from build123d import *

# Parameters (mm, degrees)
SKIZZE1_W                       = 72
SKIZZE1_H                       = 44.2
SKIZZE1_R                       = 10
SKIZZE1_R_2                     = 6
AUFSATZ_LINEAR_AUSTRAGEN1_DEPTH = 20
FASE1_SIZE                      = 10
FASE2_SIZE                      = 10
FASE6_SIZE                      = 10
FASE6_SIZE2                     = 3.639702343
FASE7_SIZE                      = 5
SKIZZE3_W                       = 5
SKIZZE3_H                       = 17
SCHNITT_LINEAR_AUSTRAGEN1_DEPTH = 80
SKIZZE11_R                      = 12
SCHNITT_LINEAR_AUSTRAGEN2_DEPTH = 3.4
M5_GEWINDEBOHRUNG1_D            = 4.2
M5_GEWINDEBOHRUNG1_DEPTH        = 12
M5_GEWINDEBOHRUNG1_TIP          = 1.2618073


with BuildPart() as part:
    # Skizze1 → Aufsatz-Linear austragen1 (new body)
    with BuildSketch(Plane.XY):
        with Locations((53.961300324, 0)):
            Rectangle(SKIZZE1_W, SKIZZE1_H)
        with Locations((53.961300324, -9.9)):
            Circle(SKIZZE1_R, mode=Mode.SUBTRACT)
        with Locations((33.961300324, -9.9)):
            Circle(SKIZZE1_R_2, mode=Mode.SUBTRACT)
        with Locations((73.961300324, -9.9)):
            Circle(SKIZZE1_R_2, mode=Mode.SUBTRACT)
    extrude(amount=AUFSATZ_LINEAR_AUSTRAGEN1_DEPTH)

    # Fase1
    fase1_edges = [part.edges().sort_by_distance(p)[0] for p in [
        (17.961300324, -22.1, 10),
    ]]
    chamfer(fase1_edges, length=FASE1_SIZE)

    # Fase2
    fase2_edges = [part.edges().sort_by_distance(p)[0] for p in [
        (89.961300324, -22.1, 10),
    ]]
    chamfer(fase2_edges, length=FASE2_SIZE)

    # Fase6
    fase6_edges = [part.edges().sort_by_distance(p)[0] for p in [
        (53.961300324, 22.1, 0),
    ]]
    fase6_side = [part.faces().sort_by_distance(p)[0] for p in [
        (53.961300324, 22.1, 10),
    ]]
    chamfer(fase6_edges, length=FASE6_SIZE, length2=FASE6_SIZE2, reference=fase6_side[0])

    # Fase7
    fase7_edges = [part.edges().sort_by_distance(p)[0] for p in [
        (89.961300324, 3.180148829, 0),
        (17.961300324, 3.180148829, 0),
    ]]
    chamfer(fase7_edges, length=FASE7_SIZE)

    # Skizze3 → Schnitt-Linear austragen1 (cut)
    with BuildSketch(Plane.ZY.offset(-17.961300324)):
        with Locations((17.5, 13.6)):
            Rectangle(SKIZZE3_W, SKIZZE3_H)
    extrude(amount=-SCHNITT_LINEAR_AUSTRAGEN1_DEPTH, mode=Mode.SUBTRACT)

    # Skizze11 → Schnitt-Linear austragen2 (cut)
    with BuildSketch(Plane(origin=(0, 0, 0), x_dir=(-1, 0, 0), z_dir=(0, 0, -1))):
        with Locations((-53.961300324, -9.9)):
            Circle(SKIZZE11_R)
    extrude(amount=-SCHNITT_LINEAR_AUSTRAGEN2_DEPTH, mode=Mode.SUBTRACT)

    # M5 Gewindebohrung1
    with Locations(Plane.XY.offset(15)):
        with Locations((31.282727226, 13.273175205), (79.505567547, 13.273175205)):
            Hole(M5_GEWINDEBOHRUNG1_D / 2, depth=M5_GEWINDEBOHRUNG1_DEPTH)
            with Locations((0, 0, -(M5_GEWINDEBOHRUNG1_DEPTH + M5_GEWINDEBOHRUNG1_TIP / 2))):  # 118° drill point
                Cone(0, M5_GEWINDEBOHRUNG1_D / 2, M5_GEWINDEBOHRUNG1_TIP, mode=Mode.SUBTRACT)


solid = part.part
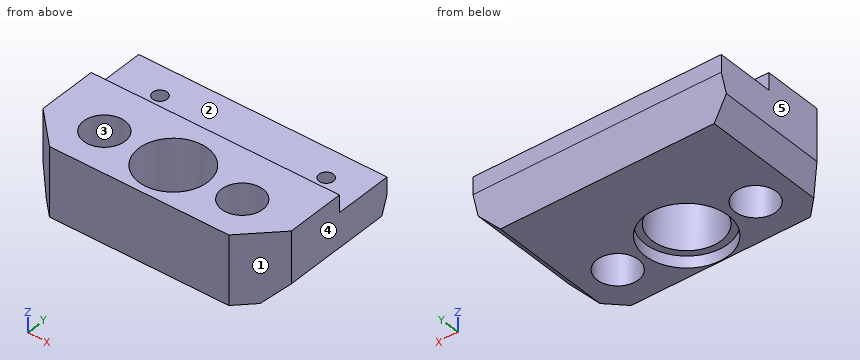
Input: part model. Units: mm. Frame: model coordinates. Face numbers are marked on the shaded views. A direction names the side the tool comes from. Give positions to 0.01 mm unless a question says otherwise; leave off trailing zeros. Loops run counter-clockwise (first coordinate to the right, second up) from the corner with the lowest first, then second, coordinate; pieces in that order, holes last. Notation, with made-up numbers: M 0,22.5 L 34,22.5 A22 ccw 34,28.5 Z; hole C 77,5.5 d7. An arc over 180 degrees is marked long. Use one line per item in the form item = value.
1. Pull-direction query (X, two-part tool) for the marked faces 3, 4 and 5; classes: released by +X, released by -X, zero draft, split by the parting line, or undercut.
Numbers:
face_3 = undercut
face_4 = released by +X
face_5 = released by -X
2. First-contact query: pin 1 (12 mm diameter, centred on x = 81, y = 17.5, fed in from +Z); pin 2 (5 mm diameter, centred on y = -13.5, z = 2.5, fed in from -X); pin 3 (7 mm diameter, centred on x = 33.96, y = -9.9, fed in from -Z); pin 4 (2 mm diameter, centred on x = 68.5, y = -8, fed in from +Z). Flat tips, straight axial feed; report the tip coordinate or a pass-through.
Numbers:
pin_1 = 15
pin_2 = 18.23
pin_3 = through
pin_4 = 20
3. Line query: L1, parallel to X at y = -9.5, z = 16.75; L2, parallel to X at y = 11.5, z = 7.75; L3, parallel to X at y = -12.5, z = 15. Output: solid intervals per line, ascending.
Numbers:
L1 = 17.96 to 27.97, 39.95 to 43.97, 63.95 to 67.97, 79.95 to 89.96
L2 = 17.96 to 30.16, 32.41 to 78.38, 80.63 to 89.96
L3 = 18.36 to 28.55, 39.37 to 44.31, 63.62 to 68.55, 79.37 to 89.56
4. Reachability of the marked faces 1 and 2 from +Z, -Z, +X, -X, +Y, -Y: full face, straight path, thin tool, end or side. Return the list, or none.
Numbers:
face_1 = +Z, -Z, +X, -Y
face_2 = +Z, +X, -X, +Y
5. Section query C-C, the plane z = 7. Return the cut outline in (x, y).
Numbers:
outline = M 17.96,-12.1 L 27.96,-22.1 L 79.96,-22.1 L 89.96,-12.1 L 89.96,21.01 L 17.96,21.01 Z; hole C 33.96,-9.9 d12; hole C 31.28,13.27 d4.2; hole C 53.96,-9.9 d20; hole C 73.96,-9.9 d12; hole C 79.51,13.27 d4.2
6. Section query B-B, the plane y = -2. Return the cut outline in (x, z).
Numbers:
outline = M 17.96,5 L 22.96,0 L 44.93,0 L 44.93,3.4 L 47.83,3.4 L 47.83,20 L 17.96,20 Z; M 60.09,3.4 L 62.99,3.4 L 62.99,0 L 84.96,0 L 89.96,5 L 89.96,20 L 60.09,20 Z
7. Section query A-A, the plane y = -9.9. Return the cut outline in (x, z), and give its area (3 significant figures).
Numbers:
outline = M 17.96,5 L 22.96,0 L 27.96,0 L 27.96,20 L 17.96,20 Z; M 39.96,0 L 41.96,0 L 41.96,3.4 L 43.96,3.4 L 43.96,20 L 39.96,20 Z; M 63.96,3.4 L 65.96,3.4 L 65.96,0 L 67.96,0 L 67.96,20 L 63.96,20 Z; M 79.96,0 L 84.96,0 L 89.96,5 L 89.96,20 L 79.96,20 Z
area = 521 mm²
